Design review of the part built by this model. Coordinates are the model's own, in mm. A direction names the side the tool comes from. Give positions to 0.01 mm unless a question says otherwise; leave off trailing zeros. Write each loop counter-clockwise with the first axis right and the second up, starting at its lowest first coordinate (ties: lowest second). Pieces come first, ordered by that corner, then holes. Notation, with made-up numbers: M 79,-35.75 L 132,-35.75 A16 ccw 132,-23.75 Z; hole C 21,-9 d5. An arc over 180 degrees is marked long. Answer in a Markdown table with one row per item.
```python
from build123d import *

# Parameters (mm, degrees)
F0_W     = 19.05
F0_H     = 12.7
F1_DEPTH = 31.75
F2_W     = 6.35
F2_H     = 6.35
F3_DEPTH = 31.75
F5_DEPTH = 50.8
F6_R     = 3.175
F7_DEPTH = 31.697754
F8_R     = 3.175
F9_DEPTH = 25.4


with BuildPart() as f1:
    # F0 (on Right) → F1 (new body)
    with BuildSketch(Plane.YZ):
        with Locations((9.525, -6.35)):
            Rectangle(F0_W, F0_H)
    extrude(amount=F1_DEPTH)

    # F2 (on face) → F3 (join)
    with BuildSketch(Plane.YZ.offset(31.75)):
        with Locations((15.875, -15.875)):
            Rectangle(F2_W, F2_H)
    extrude(amount=-F3_DEPTH)

    # F4 (on face) → F5 (join)
    with BuildSketch(Plane.YZ.offset(31.75)):
        Polygon((19.05, -19.05), (12.7, -19.05), (12.7, -31.696754), (25.4, -31.696754), (25.4, -25.346754), (19.05, -25.4), align=None)
    extrude(amount=-F5_DEPTH)

    # F6 (on face) → F7 (cut, through all)
    with BuildSketch(Plane.XY):
        with Locations((6.35, 6.35)):
            Circle(F6_R)
    extrude(amount=-F7_DEPTH, mode=Mode.SUBTRACT)

    # F8 (on face) → F9 (cut)
    with BuildSketch(Plane(origin=(0, 19.05, 0), x_dir=(-1, 0, 0), z_dir=(0, 1, 0))):
        with Locations((-22.098, -6.35)):
            Circle(F8_R)
    extrude(amount=-F9_DEPTH, mode=Mode.SUBTRACT)


solid = f1.part
```
1) Add section C-C (y = 16.5). Write out the cut boundary in (x, z) (3 decimals), and give its area (3 significant figures).
Geometry says:
| item | result |
|---|---|
| outline | M -19.05,-31.697 L 31.75,-31.697 L 31.75,0 L 0,0 L 0,-19.05 L -19.05,-19.05 Z; hole C 22.098,-6.35 d6.35 |
| area | 1,220 mm^2 |
2) Add section A-A (z = -6.35). Write out the cut boundary in (x, y) (3 decimals).
Geometry says:
| item | result |
|---|---|
| outline | M 0,0 L 18.923,0 L 18.923,19.05 L 0,19.05 Z; M 25.273,0 L 31.75,0 L 31.75,19.05 L 25.273,19.05 Z; hole C 6.35,6.35 d6.35 |
3) For faces 5 (the face through (22.79, 9.66, -9.45)), 6 (the face through (0, 9, -7)), 7 (the face through (16, 6, -12.7)), list the 3-axis set-ups (+Z, -Z, +X, -X, +Y, -Y) from which the entire face can be reached by the end or side of a thin tool; tool diameter is ignored.
Geometry says:
| item | result |
|---|---|
| face 5 | +Y, -Y |
| face 6 | +Z, -X, +Y, -Y |
| face 7 | -Z, +X, -X, -Y |
4) To check wall thickness, follow probe 1 along Y at (x, z) = (6.35, -7.5) (3 decimals); probe 2 along Y at (x, z) = (5, -28); probe 3 along Z at (x, y) = (20, 12.5). State the ranges of each line that lie inside material, in increasing order. Write a range as [from, to].
Geometry says:
| item | result |
|---|---|
| probe 1 | [0, 3.175], [9.525, 19.05] |
| probe 2 | [12.7, 25.4] |
| probe 3 | [-12.7, -8.73], [-3.97, 0] |
5) Add section D-D (y = 8.5). Write out the cut boundary in (x, z) (3 decimals).
Geometry says:
| item | result |
|---|---|
| outline | M 0,-12.7 L 4.014,-12.7 L 4.014,0 L 0,0 Z; M 8.686,-12.7 L 31.75,-12.7 L 31.75,0 L 8.686,0 Z; hole C 22.098,-6.35 d6.35 |
6) Insertion check: P1, Ø4, axis at x = 9, y = 9, coming from the -Z side; P2, Ø12, axis at x = 12.5, z = -22.5, coming from the -Y side; P3, Ø5.5, axis at y = 5.5, z = -9.5, coming from the -X side. Each pin has a flat end and moves straight along its axis. Give the tip position at first contact, or say it passes through.
Geometry says:
| item | result |
|---|---|
| P1 | z = -12.7 |
| P2 | y = 12.7 |
| P3 | x = 0 |
7) The part is to be moulded in two halves that separate along Y. For faces 1 (the face through (7, 25.4, -29)), 2 (the face through (4.01, 8.496, -6.261)), 3 (the face through (-9, 16, -19.05)), 4 (the face through (7, 12.7, -22)), say which applies: released by +Y, released by -Y, zero draft, split by the parting line, or undercut.
Geometry says:
| item | result |
|---|---|
| face 1 | released by +Y |
| face 2 | undercut |
| face 3 | zero draft |
| face 4 | released by -Y |
8) Add section B-B (x = 6.35). Write out the cut boundary in (y, z) (3 decimals), and give its area (3 significant figures).
Geometry says:
| item | result |
|---|---|
| outline | M 0,-12.7 L 3.175,-12.7 L 3.175,0 L 0,0 Z; M 9.525,-12.7 L 12.7,-12.7 L 12.7,-31.697 L 25.4,-31.697 L 25.4,-25.347 L 19.05,-25.4 L 19.05,0 L 9.525,0 Z |
| area | 322 mm^2 |
